```python
from build123d import *

# Parameters (mm, degrees)
SKETCH_1_R           = 1.5
EXTRUDE_1_DEPTH      = 8
SKETCH_2_W           = 17
SKETCH_2_H           = 26.3
CUT_EXTRUDE_1_DEPTH  = 4.4
CUT_EXTRUDE_3_DEPTH  = 5.5
CUT_EXTRUDE_4_DEPTH  = 3.5
CUT_EXTRUDE_5_DEPTH  = 3.5
SKETCH_9_R           = 1.25
CUT_EXTRUDE_6_DEPTH  = 6
SKETCH_10_R          = 1.25
CUT_EXTRUDE_7_DEPTH  = 6
SKETCH_11_R          = 1.25
CUT_EXTRUDE_8_DEPTH  = 6
SKETCH_12_R          = 1.25
CUT_EXTRUDE_9_DEPTH  = 6
SKETCH_13_R          = 1
SKETCH_13_R_2        = 1.25
CUT_EXTRUDE_10_DEPTH = 46


with BuildPart() as part:
    # Эскиз1 → Бобышка-Вытянуть1 (new body)
    with BuildSketch(Plane(origin=(0, 0, 0), x_dir=(1, 0, 0), z_dir=(0, 1, 0))):
        Polygon((-23, 16.5), (23, 16.5), (23, 13.15), (54.5, 13.15), (54.5, -13.15), (23, -13.15), (23, -16.5), (-23, -16.5), (-23, -13.15), (-31, -13.15), (-31, 13.15), (-23, 13.15), align=None)
        with Locations(Location((40.5, 7.15, 0), (0, 0, 270))):  # turned: the seam where the file's is
            Circle(SKETCH_1_R, mode=Mode.SUBTRACT)
        with Locations(Location((40.5, -7.15, 0), (0, 0, 90))):  # turned: the seam where the file's is
            Circle(SKETCH_1_R, mode=Mode.SUBTRACT)
    extrude(amount=EXTRUDE_1_DEPTH)

    # Эскиз2 → Вырез-Вытянуть1 (cut)
    with BuildSketch(Plane(origin=(0, 8, 0), x_dir=(1, 0, 0), z_dir=(0, 1, 0))):
        with Locations((46, 0)):
            Rectangle(SKETCH_2_W, SKETCH_2_H)
    extrude(amount=-CUT_EXTRUDE_1_DEPTH, mode=Mode.SUBTRACT)

    # Эскиз3 → Вырез-Вытянуть3 (cut)
    with BuildSketch(Plane(origin=(0, 8, 0), x_dir=(1, 0, 0), z_dir=(0, 1, 0))):
        with BuildLine():
            Line((-25.795194039, -8), (-12, -8))
            Line((-12, -8), (-12, -12.295194039))
            ThreePointArc((-12, -12.295194039), (-11.354227285, -13.854227285), (-9.795194039, -14.5))
            Line((-9.795194039, -14.5), (18.795194039, -14.5))
            ThreePointArc((18.795194039, -14.5), (20.354227285, -13.854227285), (21, -12.295194039))
            Line((21, -12.295194039), (21, -8))
            Line((21, -8), (32.295194039, -8))
            ThreePointArc((32.295194039, -8), (33.854227285, -7.354227285), (34.5, -5.795194039))
            Line((34.5, -5.795194039), (34.5, 5.795194039))
            ThreePointArc((34.5, 5.795194039), (33.854227285, 7.354227285), (32.295194039, 8))
            Line((32.295194039, 8), (21, 8))
            Line((21, 8), (21, 12.295194039))
            ThreePointArc((21, 12.295194039), (20.354227285, 13.854227285), (18.795194039, 14.5))
            Line((18.795194039, 14.5), (-9.795194039, 14.5))
            ThreePointArc((-9.795194039, 14.5), (-11.354227285, 13.854227285), (-12, 12.295194039))
            Line((-12, 12.295194039), (-12, 8))
            Line((-12, 8), (-25.795194039, 8))
            ThreePointArc((-25.795194039, 8), (-27.354227285, 7.354227285), (-28, 5.795194039))
            Line((-28, 5.795194039), (-28, -5.795194039))
            ThreePointArc((-28, -5.795194039), (-27.354227285, -7.354227285), (-25.795194039, -8))
        make_face()
    extrude(amount=-CUT_EXTRUDE_3_DEPTH, mode=Mode.SUBTRACT)

    # Эскиз6 → Вырез-Вытянуть4 (cut, through all)
    with BuildSketch(Plane(origin=(0, 2.5, 0), x_dir=(1, 0, 0), z_dir=(0, 1, 0))):
        with BuildLine():
            Line((-7, 2), (-7, -2))
            ThreePointArc((-7, -2), (-4.949747468, -6.949747468), (0, -9))
            Line((0, -9), (8, -9))
            ThreePointArc((8, -9), (12.949747468, -6.949747468), (15, -2))
            Line((15, -2), (15, 2))
            ThreePointArc((15, 2), (12.949747468, 6.949747468), (8, 9))
            Line((8, 9), (0, 9))
            ThreePointArc((0, 9), (-4.949747468, 6.949747468), (-7, 2))
        make_face()
    extrude(amount=-CUT_EXTRUDE_4_DEPTH, mode=Mode.SUBTRACT)

    # Эскиз7 → Вырез-Вытянуть5 (cut, through all)
    with BuildSketch(Plane(origin=(0, 2.5, 0), x_dir=(1, 0, 0), z_dir=(0, 1, 0))):
        with BuildLine():
            Line((12.5, 12.5), (16.5, 12.5))
            ThreePointArc((16.5, 12.5), (18.5, 10.5), (16.5, 8.5))
            Line((16.5, 8.5), (12.5, 8.5))
            ThreePointArc((12.5, 8.5), (10.5, 10.5), (12.5, 12.5))
        make_face()
        with BuildLine():
            Line((-4.5, 8.5), (-8.5, 8.5))
            ThreePointArc((-8.5, 8.5), (-10.5, 10.5), (-8.5, 12.5))
            Line((-8.5, 12.5), (-4.5, 12.5))
            ThreePointArc((-4.5, 12.5), (-2.5, 10.5), (-4.5, 8.5))
        make_face()
        with BuildLine():
            Line((12.5, -8.5), (16.5, -8.5))
            ThreePointArc((16.5, -8.5), (18.5, -10.5), (16.5, -12.5))
            Line((16.5, -12.5), (12.5, -12.5))
            ThreePointArc((12.5, -12.5), (10.5, -10.5), (12.5, -8.5))
        make_face()
        with BuildLine():
            Line((-4.5, -8.5), (-8.5, -8.5))
            ThreePointArc((-8.5, -8.5), (-10.5, -10.5), (-8.5, -12.5))
            Line((-8.5, -12.5), (-4.5, -12.5))
            ThreePointArc((-4.5, -12.5), (-2.5, -10.5), (-4.5, -8.5))
        make_face()
    extrude(amount=-CUT_EXTRUDE_5_DEPTH, mode=Mode.SUBTRACT)

    # Эскиз9 → Вырез-Вытянуть6 (cut)
    with BuildSketch(Plane.XY.offset(13.15)):
        with Locations((-27, 4)):
            Circle(SKETCH_9_R)
    extrude(amount=-CUT_EXTRUDE_6_DEPTH, mode=Mode.SUBTRACT)

    # Эскиз10 → Вырез-Вытянуть7 (cut)
    with BuildSketch(Plane(origin=(0, 0, -13.15), x_dir=(-1, 0, 0), z_dir=(0, 0, -1))):
        with Locations(Location((27, 4, 0), (0, 0, 180))):  # turned: the seam where the file's is
            Circle(SKETCH_10_R)
    extrude(amount=-CUT_EXTRUDE_7_DEPTH, mode=Mode.SUBTRACT)

    # Эскиз11 → Вырез-Вытянуть8 (cut)
    with BuildSketch(Plane(origin=(0, 0, -13.15), x_dir=(-1, 0, 0), z_dir=(0, 0, -1))):
        with Locations((-27, 4)):
            Circle(SKETCH_11_R)
    extrude(amount=-CUT_EXTRUDE_8_DEPTH, mode=Mode.SUBTRACT)

    # Эскиз12 → Вырез-Вытянуть9 (cut)
    with BuildSketch(Plane.XY.offset(13.15)):
        with Locations(Location((27, 4, 0), (0, 0, 180))):  # turned: the seam where the file's is
            Circle(SKETCH_12_R)
    extrude(amount=-CUT_EXTRUDE_9_DEPTH, mode=Mode.SUBTRACT)

    # Эскиз13 → Вырез-Вытянуть10 (cut)
    with BuildSketch(Plane.XY.offset(16.5)):
        with Locations((-5, 4)):
            Circle(SKETCH_13_R)
        with Locations((-14.5, 4)):
            Circle(SKETCH_13_R_2)
    extrude(amount=-CUT_EXTRUDE_10_DEPTH, mode=Mode.SUBTRACT)


solid = part.part
```
Part model, mm, in its own coordinate system. A direction names the side the tool comes from. Round coordinates to 2 decimals unless told otherwise and drop trailing zeros. Order: outer loops, then holes, each group sorted by start corner. A loop starts at its lowest first (then second) coordinate and runs counter-clockwise, first axis right, second up. Notation, with made-up numbers: M 19,69 L 66,69 A18 ccw 66,101 Z; hole C 39,-35.5 d11. An arc over 180 degrees is marked long. Put each result on its own line as item: value. Start each with the question number.
1. Slice it at D-D on x = 22. List the corners of the cut face in (y, z), then the cut area to 3 significant figures.
2. Drill centre lines: probe 1 along Z at (x, y) = (-1.5, 3.25); probe 2 along X at (y, z) = (3.5, -5); probe 3 along X at (y, z) = (4.25, -2). Where is each one in solid material? Low to high. Write a range as [from, to].
3. Tool access for faces 4 (the face through (-31, 4, 0)), 5 (the face through (-23, 4, 15)), 6 (the face through (34.5, 5, 0)), 7 (the face through (13, 1.3, -6.9)): list every direction of +Z, -Z, +X, -X, +Y, -Y with a clear straight run to the whole face (end or side of a thin tool).
4. Two-plate mould, pull along Z, no slides. Class faces 1 (the face through (-5, 5, 16)), 2 (the face through (-6, 1, -8.5)), 3 (the face through (35, 3, -13.15)): +Z half, -Z half, draft (parallel to the pull), parting line (faces both ways), or undercut.
5. Slice it at A-A on z = 10.5. List the corners of the cut face in (x, y), then the cut area to 3 significant figures.
6. Drop flat-ended pins along their axis: pin 1 (3.5 mm diameter, centred on y = 6, z = 10.5, fed in from +X); pin 2 (13.5 mm diameter, centred on x = 44.5, z = -2, fed in from +Y); pin 3 (3 mm diameter, centred on x = 26, y = 4.5, fed in from -Z); pin 4 (1 mm diameter, centred on x = -3.5, z = -6.5, fed in from +Y). Give the stop position or say it passes through.
7. Slice it at C-C on z = -1. List the corners of the cut face in (x, y).
8. Slice it at B-B on x = 40.5. List the corners of the cut face in (y, z), then the cut area to 3 significant figures.
Findings:
1. outline: M 0,-16.5 L 8,-16.5 L 8,-8 L 2.5,-8 L 2.5,8 L 8,8 L 8,16.5 L 0,16.5 Z
1. area: 176 mm2
2. probe 1: [-16.5, -14.5], [14.5, 16.5]
2. probe 2: [-31, -28], [34.5, 54.5]
2. probe 3: [-31, -28], [34.5, 37.5]
3. face 4: +Z, -Z, -X, +Y, -Y
3. face 5: +Z, -X, +Y, -Y
3. face 6: +Y
3. face 7: +Y, -Y
4. face 1: draft
4. face 2: undercut
4. face 3: -Z half
5. outline: M -31,0 L -10.5,0 L -10.5,2.5 L -12,2.5 L -12,8 L -31,8 Z; M -2.5,0 L 10.5,0 L 10.5,2.5 L -2.5,2.5 Z; M 18.5,0 L 54.5,0 L 54.5,3.6 L 37.5,3.6 L 37.5,8 L 21,8 L 21,2.5 L 18.5,2.5 Z; hole C -27,4 d2.5; hole C -14.5,4 d2.5; hole C 27,4 d2.5
5. area: 373 mm2
6. pin 1: x = 37.5
6. pin 2: y = 3.6
6. pin 3: z = -13.15
6. pin 4: through
7. outline: M -31,0 L -7,0 L -7,2.5 L -28,2.5 L -28,8 L -31,8 Z; M 15,0 L 54.5,0 L 54.5,3.6 L 37.5,3.6 L 37.5,8 L 34.5,8 L 34.5,2.5 L 15,2.5 Z
8. outline: M 0,-13.15 L 3.6,-13.15 L 3.6,-8.65 L 0,-8.65 Z; M 0,-5.65 L 3.6,-5.65 L 3.6,5.65 L 0,5.65 Z; M 0,8.65 L 3.6,8.65 L 3.6,13.15 L 0,13.15 Z
8. area: 73.1 mm2
